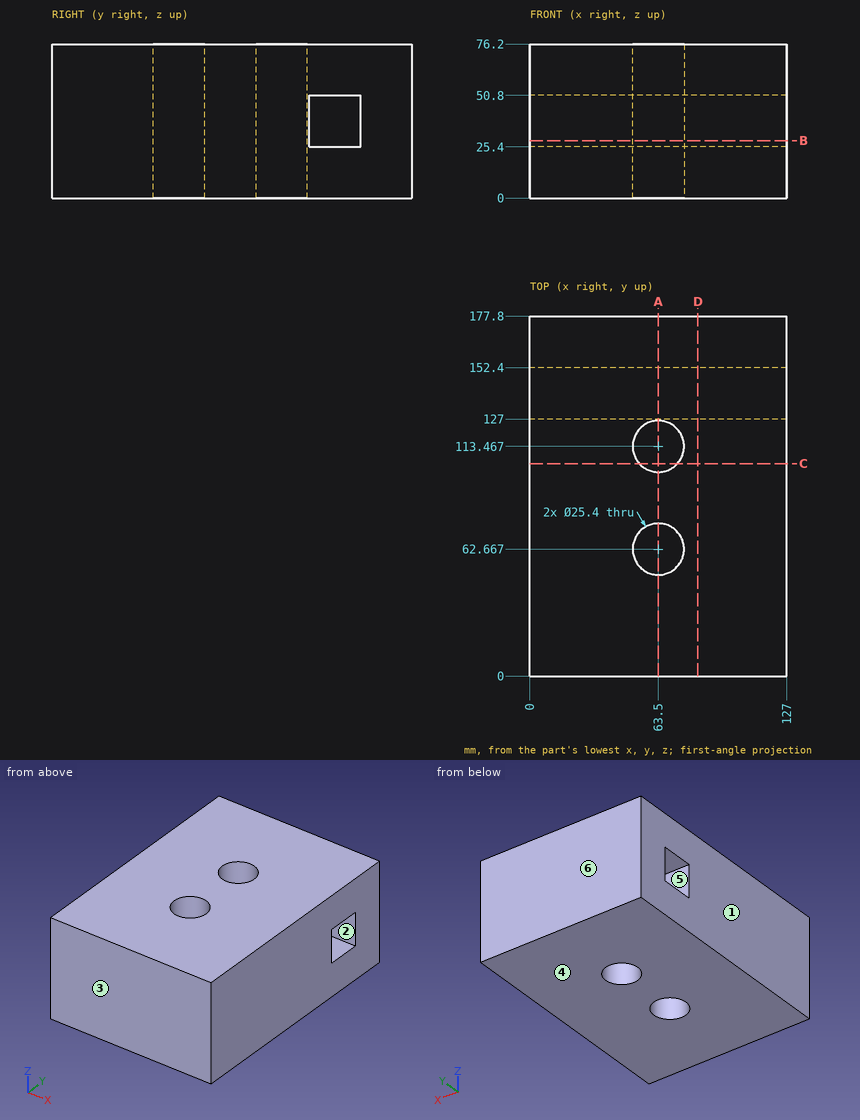
Drawing for the job (mm, zero at the part's lowest x, y, z). A direction names the side the tool comes from. Round coordinates to 2 decimals unless told otherwise and drop trailing zeros. Write each loop counter-clockwise with the first axis right and the second up, starting at its lowest first coordinate (ties: lowest second). Pieces come first, ordered by that corner, then holes. Notation, with made-up numbers: (30, 56.25) - (70, 56.25) arc R18 cw to (70, 68.25) - close; hole circle Ø2 at (73.5, -39.5). An arc over 180 degrees is marked (long way). Write item = value, one per line. Start each with the question number.
Q1. Mould opens along Y. For the marked faces 3, 4, 5 and 6 say: pulls with the +Y half, pulls with the -Y half, needs draft (parallel to the pull), parting line crosses it, or undercut.
Q2. Band-saw the part on B-B (z = 28.5). Give the cut face in (x, y), then the cut area to 3 significant figures.
Q3. Band-saw the part on C-C (y = 105). Give the cut face in (x, z) (1 decimal).
Q4. Which spindle directions (+Z, -Z, +X, -X, +Y, -Y) get a long thin tool onto all of the face, cutting with end or side? Do the marked faces 1 and 2. Say none if no direction does.
Q5. Band-saw the part on D-D (x = 83). Give the cut face in (y, z), then the cut area to 3 significant figures.
Q6. Probe L1, parallel to Y at x = 63.5, z = 23.5; L2, parallel to Y at x = 63, z = 33; L3, parallel to Y at x = 30.5, z = 47. List the from-to ranges inside material, lowest first. Write a range as from..to.
Q7. Band-saw the part on A-A (x = 63.5). Give the cut face in (y, z).
Answers below:
q1.face_3 = pulls with the -Y half
q1.face_4 = needs draft
q1.face_5 = undercut
q1.face_6 = pulls with the +Y half
q2.outline = (0, 0) - (127, 0) - (127, 127) - (0, 127) - close; (0, 152.4) - (127, 152.4) - (127, 177.8) - (0, 177.8) - close; hole circle Ø25.4 at (63.5, 62.67); hole circle Ø25.4 at (63.5, 113.47)
q2.area = 18,300 mm2
q3.outline = (0, 0) - (54, 0) - (54, 76.2) - (0, 76.2) - close; (73, 0) - (127, 0) - (127, 76.2) - (73, 76.2) - close
q4.face_1 = +Z, -Z, -X, +Y, -Y
q4.face_2 = +X, -X
q5.outline = (0, 0) - (177.8, 0) - (177.8, 76.2) - (0, 76.2) - close; hole (127, 25.4) - (152.4, 25.4) - (152.4, 50.8) - (127, 50.8) - close
q5.area = 12,900 mm2
q6.L1 = 0..49.97, 75.37..100.77, 126.17..177.8
q6.L2 = 0..49.98, 75.36..100.78, 126.16..127, 152.4..177.8
q6.L3 = 0..127, 152.4..177.8
q7.outline = (0, 0) - (49.97, 0) - (49.97, 76.2) - (0, 76.2) - close; (75.37, 0) - (100.77, 0) - (100.77, 76.2) - (75.37, 76.2) - close; (126.17, 0) - (177.8, 0) - (177.8, 76.2) - (126.17, 76.2) - close; hole (127, 25.4) - (152.4, 25.4) - (152.4, 50.8) - (127, 50.8) - close
